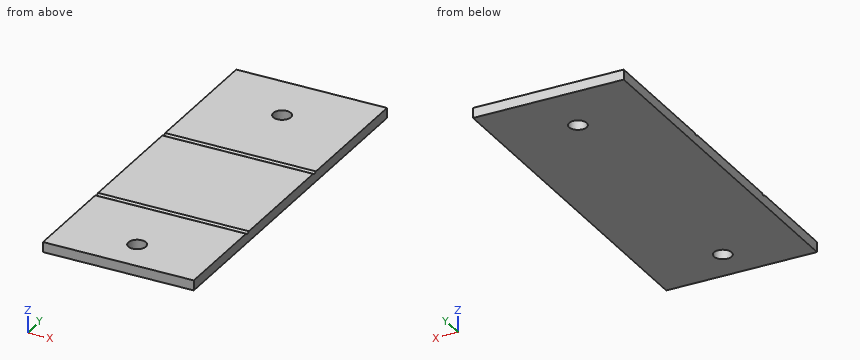
```python
from build123d import *

# Parameters (mm, degrees)
F0_W     = 30
F0_H     = 27
F0_R     = 1.75
F0_H_2   = 25
F0_H_3   = 20
F1_DEPTH = 2
F3_DEPTH = 30.001


with BuildPart() as f1:
    # F0 (on Top) → F1 (new body)
    with BuildSketch(Plane.XY):
        with Locations((15, 58.5)):
            Rectangle(F0_W, F0_H)
        with Locations((15, 61)):
            Circle(F0_R, mode=Mode.SUBTRACT)
        with Locations((15, 32.5)):
            Rectangle(F0_W, F0_H_2)
        with Locations((15, 10)):
            Rectangle(F0_W, F0_H_3)
        with Locations((15, 7)):
            Circle(F0_R, mode=Mode.SUBTRACT)
    extrude(amount=F1_DEPTH)

    # F2 (on face) → F3 (cut, through all)
    with BuildSketch(Plane(origin=(0, 0, 0), x_dir=(0, -1, 0), z_dir=(-1, 0, 0))):
        Polygon((-20, 1.7), (-19.480385, 2), (-20.519615, 2), align=None)
        Polygon((-44.480385, 2), (-45.519615, 2), (-45, 1.7), align=None)
    extrude(amount=-F3_DEPTH, mode=Mode.SUBTRACT)


solid = f1.part
```
The listing builds one solid part. Answer for the finished solid, in the listing's coordinates (mm). Coordinates: 2 decimals unless noted, no trailing zeros. Write each loop counter-clockwise with the first axis right and the second up, starting at its lowest first coordinate (ties: lowest second). Pieces come first, ordered by that corner, then holes. Notation, with made-up numbers: (25, -14.75) - (69, -14.75) arc R22 ccw to (69, 15.25) - close; hole circle Ø8 at (15.25, -6). An arc over 180 degrees is marked (long way). Return JSON: item names as keys, results as strings. Group by question number.
1. Straight lines are drawn through the part: L1, parallel to Y at x = 15, z = 0.9; L2, parallel to Y at x = 18.75, z = 1.8; L3, parallel to X at y = 59.5, z = 1.8. For each, find the intervals that lie inside material, in ascending order.
2. A cutting plane is placed at B-B, the plane x = 15. Determine the outline of the cut face in (y, z), plus the area to 3 significant figures.
3. A cutting plane is placed at A-A, the plane y = 61. Determine the outline of the cut face in (x, z).
Ans:
{
 "1": {"L1": "0 to 5.25, 8.75 to 59.25, 62.75 to 72", "L2": "0 to 19.83, 20.17 to 44.83, 45.17 to 72", "L3": "0 to 14.1, 15.9 to 30"},
 "2": {"outline": "(0, 0) - (5.25, 0) - (5.25, 2) - (0, 2) - close; (8.75, 0) - (59.25, 0) - (59.25, 2) - (45.52, 2) - (45, 1.7) - (44.48, 2) - (20.52, 2) - (20, 1.7) - (19.48, 2) - (8.75, 2) - close; (62.75, 0) - (72, 0) - (72, 2) - (62.75, 2) - close", "area": "130 mm²"},
 "3": {"outline": "(0, 0) - (13.25, 0) - (13.25, 2) - (0, 2) - close; (16.75, 0) - (30, 0) - (30, 2) - (16.75, 2) - close"}
}
